```python
from build123d import *

# Parameters (mm, degrees)
SKETCH2_W                 = 114.3
SKETCH2_H                 = 101.6
BOSS_EXTRUDE2_DEPTH       = 19.05
M8X1_0_TAPPED_HOLE1_D     = 7
M8X1_0_TAPPED_HOLE1_DEPTH = 19.05
M8X1_0_TAPPED_HOLE1_TIP   = 2.103012167
M8X1_0_TAPPED_HOLE2_D     = 7
M8X1_0_TAPPED_HOLE2_DEPTH = 19.05
M8X1_0_TAPPED_HOLE2_TIP   = 2.103012167
SKETCH7_R                 = 23.5000038
CUT_EXTRUDE1_DEPTH        = 13.99999994
CUT_EXTRUDE5_DEPTH        = 5.08


with BuildPart() as part:
    # Sketch2 → Boss-Extrude2 (new body)
    with BuildSketch(Plane(origin=(0, 0, 0), x_dir=(0, 1, 0), z_dir=(0, 0, 1))):
        with Locations((57.15, 50.8)):
            Rectangle(SKETCH2_W, SKETCH2_H)
    extrude(amount=BOSS_EXTRUDE2_DEPTH)

    # M8x1.0 Tapped Hole1
    with Locations(Plane.XZ):
        with Locations((-28.448, 9.652), (-73.152, 9.652)):
            Hole(M8X1_0_TAPPED_HOLE1_D / 2, depth=M8X1_0_TAPPED_HOLE1_DEPTH)
            with Locations((0, 0, -(M8X1_0_TAPPED_HOLE1_DEPTH + M8X1_0_TAPPED_HOLE1_TIP / 2))):  # 118° drill point
                Cone(0, M8X1_0_TAPPED_HOLE1_D / 2, M8X1_0_TAPPED_HOLE1_TIP, mode=Mode.SUBTRACT)

    # M8x1.0 Tapped Hole2
    with Locations(Plane(origin=(0, 114.3, 0), x_dir=(-1, 0, 0), z_dir=(0, 1, 0))):
        with Locations((73.152, 9.398), (28.448, 9.398)):
            Hole(M8X1_0_TAPPED_HOLE2_D / 2, depth=M8X1_0_TAPPED_HOLE2_DEPTH)
            with Locations((0, 0, -(M8X1_0_TAPPED_HOLE2_DEPTH + M8X1_0_TAPPED_HOLE2_TIP / 2))):  # 118° drill point
                Cone(0, M8X1_0_TAPPED_HOLE2_D / 2, M8X1_0_TAPPED_HOLE2_TIP, mode=Mode.SUBTRACT)

    # Sketch7 → Cut-Extrude1 (cut)
    with BuildSketch(Plane.XY.offset(19.05)):
        with Locations((-50.8, 57.15)):
            Circle(SKETCH7_R)
    extrude(amount=-CUT_EXTRUDE1_DEPTH, mode=Mode.SUBTRACT)

    # Sketch8 → Cut-Extrude5 (cut)
    with BuildSketch(Plane(origin=(0, 0, 0), x_dir=(1, 0, 0), z_dir=(0, 0, -1))):
        with BuildLine():
            Line((-40.64, -33.6499962), (-40.64, -80.6500038))
            ThreePointArc((-40.64, -80.6500038), (-50.8, -90.8100038), (-60.96, -80.6500038))
            Line((-60.96, -80.6500038), (-60.96, -33.6499962))
            ThreePointArc((-60.96, -33.6499962), (-50.8, -23.4899962), (-40.64, -33.6499962))
        make_face()
    extrude(amount=-CUT_EXTRUDE5_DEPTH, mode=Mode.SUBTRACT)


solid = part.part
```
The listing builds one solid part. Answer for the finished solid, in the listing's coordinates (mm). A direction names the side the tool comes from. Give positions to 0.01 mm unless a question says otherwise; leave off trailing zeros. Order: outer loops, then holes, each group sorted by start corner. A loop starts at its lowest first (then second) coordinate and runs counter-clockwise, first axis right, second up. Notation, with made-up numbers: (31, 47.25) - (37, 47.25) arc R20 cw to (37, 63.25) - close; hole circle Ø2 at (-11, 6). An arc over 180 degrees is marked (long way). Use one line per item in the form item = value. Start each with the question number.
(1) A cutting plane is placed at D-D, the plane y = 106. Write down the section's boundary in (x, z), then the cut area to 3 significant figures.
(2) A cutting plane is placed at A-A, the plane y = 57.15. Write down the section's boundary in (x, z), then the cut area to 3 significant figures.
(3) Consider line 1 (X direction, y = 57.15, z = 12.25); line 2 (Y direction, x = -53.5, z = 9.75); line 3 (X direction, y = 35.5, z = 6). Determine where each line is inside the solid, lowest interval first. Write a range as from..to.
(4) Flat-ended cylindrical pins translate along their axes: pin 1 Ø6 at (y, z) = (82.5, 10) entering from +X; pin 2 Ø5.5 at (x, z) = (-73.152, 9.398) entering from -Y; pin 3 Ø4 at (x, y) = (-65, 61) entering from +Z; pin 4 Ø5.5 at (x, z) = (-73.152, 9.652) entering from -Y. Find the tip coordinate at first contact, or state that the pin passes through.
(5) A cutting plane is placed at B-B, the plane x = -50.8. Write down the section's boundary in (y, z).
(6) The mould has two halves that part along Y. Classify faces 6 (the cylindrical face through (-69.45, 42.85, 12.15)), 7 (the conical face through (-73.71, 93.51, 9.17)), 8 (the flat face through (-52, 31, 19.05)): released by +Y, released by -Y, zero draft, split by the parting line, or undercut.
(7) For faces 1 (the cylindrical face through (-69.655, 9.658, 9.806)), 2 (the flat face through (-50, 0, 9)), 3 (the cylindrical face through (-75.7, 104.6, 11.8)), 4 (the flat face through (-66, 57, 5.05)), 5 (the cylindrical face through (-50.577, 90.808, 2.504)), determine the directions among +Z, -Z, +X, -X, +Y, -Y from which every point of the face is accessible in a straight line to the end or side of a thin tool.
(8) A cutting plane is placed at C-C, the plane y = 29.5. Write down the section's boundary in (x, z).
Ans:
q1.outline = (-101.6, 0) - (0, 0) - (0, 19.05) - (-101.6, 19.05) - close; hole circle Ø7 at (-73.15, 9.4); hole circle Ø7 at (-28.45, 9.4)
q1.area = 1,860 mm^2
q2.outline = (-101.6, 0) - (-60.96, 0) - (-60.96, 5.05) - (-74.3, 5.05) - (-74.3, 19.05) - (-101.6, 19.05) - close; (-40.64, 0) - (0, 0) - (0, 19.05) - (-27.3, 19.05) - (-27.3, 5.05) - (-40.64, 5.05) - close
q2.area = 1,170 mm^2
q3.line_1 = -101.6..-74.3, -27.3..0
q3.line_2 = 0..33.81, 80.49..114.3
q3.line_3 = -101.6..-59.94, -41.66..0
q4.pin_1 = 0
q4.pin_2 = 19.35
q4.pin_3 = 5.05
q4.pin_4 = 19.5
q5.outline = (0, 0) - (23.49, 0) - (23.49, 5.08) - (33.65, 5.08) - (33.65, 19.05) - (0, 19.05) - close; (80.65, 5.08) - (90.81, 5.08) - (90.81, 0) - (114.3, 0) - (114.3, 19.05) - (80.65, 19.05) - close
q6.face_6 = undercut
q6.face_7 = released by +Y
q6.face_8 = zero draft
q7.face_1 = -Y
q7.face_2 = +Z, -Z, +X, -X, -Y
q7.face_3 = +Y
q7.face_4 = +Z
q7.face_5 = -Z
q8.outline = (-101.6, 0) - (-60.07, 0) - (-60.07, 5.08) - (-41.53, 5.08) - (-41.53, 0) - (0, 0) - (0, 19.05) - (-101.6, 19.05) - close
